Check sheet for the modelled part. Datum: model origin and axes. Units: mm. Give positions to 0.01 mm unless a question says otherwise; leave off trailing zeros. Answer in a Markdown table with one row per item. Add a question column.
(1) Thickness scan on L1, parallel to X at y = 34, z = -0.7; L2, parallel to X at y = -68.5, z = -1.25; L3, parallel to Y at x = -75, z = -1.15. Record the ranges inside material, lowest first.
(2) Draft check along Y on faces 1 (the face through (213.704, 0.506, -0.77)), 2 (the face through (-3, 1, -1.519)). Enter one of: released by +Y, released by -Y, zero draft, split by the parting line, or undercut.
(3) Sectioned sample at A-A on z = -0.3. State how many separate pieces and enclosed holes the cut face has, then the cut area to 3 significant figures.
(4) Go/stop test with flat-tipped pins: P1, Ø0.8, axis at x = -152, z = -1, coming from the -Y side; P2, Ø2.5, axis at x = -172.74, y = -24.84, coming from the +Z side. Record where each tip stops, or that it passes through.
from build123d import *

# Parameters (mm, degrees)
SKETCH1_W          = 463
SKETCH1_H          = 150
BASE_FLANGE1_DEPTH = 1.51892
SKETCH48_R         = 1.5
SKETCH48_R_2       = 11.5
SKETCH48_R_3       = 2.5
SKETCH48_R_4       = 2
SKETCH48_W         = 7.5
SKETCH48_H         = 45
SKETCH48_W_2       = 1.5
SKETCH48_H_2       = 4
SKETCH48_W_3       = 4
SKETCH48_H_3       = 1.5
CUT_EXTRUDE1_DEPTH = 1.51892
CUT_EXTRUDE3_DEPTH = 10


# Sheet-metal steps are written as plain solids
with BuildPart() as part:
    # Sketch1 → Base-Flange1 (new body)
    with BuildSketch(Plane.XY):
        Rectangle(SKETCH1_W, SKETCH1_H)
    extrude(amount=-BASE_FLANGE1_DEPTH)

    # Sketch48 → Cut-Extrude1 (cut)
    with BuildSketch(Plane(origin=(0, 0, -1.51892), x_dir=(-1, 0, 0), z_dir=(0, 0, -1))):
        with Locations((-186.715, -15.5)):
            Circle(SKETCH48_R)
        with Locations((-186.715, 15.5)):
            Circle(SKETCH48_R)
        with Locations((-217.715, 15.5)):
            Circle(SKETCH48_R)
        with Locations((-202.215, 0)):
            Circle(SKETCH48_R_2)
        with Locations((-217.715, -15.5)):
            Circle(SKETCH48_R)
        with Locations((-135, -7.5)):
            Circle(SKETCH48_R_3)
        with Locations((-135, -32.5)):
            Circle(SKETCH48_R_3)
        with Locations((-75, -7.5)):
            Circle(SKETCH48_R_4)
        with Locations((-75, 42.5)):
            Circle(SKETCH48_R_4)
        with Locations((135, -32.5)):
            Circle(SKETCH48_R_3)
        with Locations((135, -7.5)):
            Circle(SKETCH48_R_3)
        with Locations((75, -7.5)):
            Circle(SKETCH48_R_4)
        with Locations((75, 42.5)):
            Circle(SKETCH48_R_4)
        with Locations((172.74192, -24.83591994)):
            Circle(SKETCH48_R)
        with Locations((226.01892, -24.83591994)):
            Circle(SKETCH48_R)
        with Locations((172.74192, 67.48108)):
            Circle(SKETCH48_R)
        with Locations((226.01892, 67.48108)):
            Circle(SKETCH48_R)
        with Locations((117, -20)):
            Rectangle(SKETCH48_W, SKETCH48_H)
        with Locations((-117, -20)):
            Rectangle(SKETCH48_W, SKETCH48_H)
        with Locations((-108.75, -4)):
            Rectangle(SKETCH48_W_2, SKETCH48_H_2)
        with Locations((-125.25, -4)):
            Rectangle(SKETCH48_W_2, SKETCH48_H_2)
        with Locations((-125.25, -36)):
            Rectangle(SKETCH48_W_2, SKETCH48_H_2)
        with Locations((-108.75, -36)):
            Rectangle(SKETCH48_W_2, SKETCH48_H_2)
        with Locations((-81.5, -44.25)):
            Rectangle(SKETCH48_W_3, SKETCH48_H_3)
        with Locations((-81.5, -55.75)):
            Rectangle(SKETCH48_W_3, SKETCH48_H_3)
        with Locations((-150.75, 35)):
            Rectangle(SKETCH48_W_2, SKETCH48_H_2)
        with Locations((-162.25, 35)):
            Rectangle(SKETCH48_W_2, SKETCH48_H_2)
        with Locations((125.25, -36)):
            Rectangle(SKETCH48_W_2, SKETCH48_H_2)
        with Locations((108.75, -36)):
            Rectangle(SKETCH48_W_2, SKETCH48_H_2)
        with Locations((81.5, -44.25)):
            Rectangle(SKETCH48_W_3, SKETCH48_H_3)
        with Locations((81.5, -55.75)):
            Rectangle(SKETCH48_W_3, SKETCH48_H_3)
        with Locations((162.25, 35)):
            Rectangle(SKETCH48_W_2, SKETCH48_H_2)
        with Locations((150.75, 35)):
            Rectangle(SKETCH48_W_2, SKETCH48_H_2)
        with Locations((108.75, -4)):
            Rectangle(SKETCH48_W_2, SKETCH48_H_2)
        with Locations((125.25, -4)):
            Rectangle(SKETCH48_W_2, SKETCH48_H_2)
    extrude(amount=-CUT_EXTRUDE1_DEPTH, mode=Mode.SUBTRACT)

    # Sketch50 → Cut-Extrude3 (cut)
    with BuildSketch(Plane.XY):
        with BuildLine():
            Line((166.5, -67), (166.5, -75))
            Line((166.5, -75), (125, -75))
            Line((125, -75), (125, -67))
            ThreePointArc((125, -67), (125.585786438, -65.585786438), (127, -65))
            Line((127, -65), (164.5, -65))
            ThreePointArc((164.5, -65), (165.914213562, -65.585786438), (166.5, -67))
        make_face()
        with BuildLine():
            Line((-125, -67), (-125, -75))
            Line((-125, -75), (-166.5, -75))
            Line((-166.5, -75), (-166.5, -67))
            ThreePointArc((-166.5, -67), (-165.914213562, -65.585786438), (-164.5, -65))
            Line((-164.5, -65), (-127, -65))
            ThreePointArc((-127, -65), (-125.585786438, -65.585786438), (-125, -67))
        make_face()
    extrude(amount=-CUT_EXTRUDE3_DEPTH, mode=Mode.SUBTRACT)


solid = part.part
Reply:
| question | item | result |
|---|---|---|
| 1 | L1 | -231.5 to -163, -161.5 to -151.5, -150 to 150, 151.5 to 161.5, 163 to 231.5 |
| 1 | L2 | -231.5 to -166.5, -125 to 125, 166.5 to 231.5 |
| 1 | L3 | -75 to -9.5, -5.5 to 40.5, 44.5 to 75 |
| 2 | face 1 | undercut |
| 2 | face 2 | zero draft |
| 3 | separate pieces | 1 |
| 3 | enclosed holes | 35 |
| 3 | area | 67,300 mm^2 |
| 4 | P1 | y = -65 |
| 4 | P2 | through |
